For this review, take the finished solid that the model builds, in its own axes (mm). Give positions to 0.01 mm unless a question says otherwise; leave off trailing zeros. Write each loop counter-clockwise with the first axis right and the second up, starting at its lowest first coordinate (ties: lowest second). Pieces come first, ordered by that corner, then holes. Notation, with made-up numbers: M -22.75,-36 L 30.25,-36 A20 cw 30.25,-5 Z; hole C 44.5,84 d7. An arc over 180 degrees is marked long. One line per item, written item: value. Start each with the question number.
Item 1: To check wall thickness, follow probe 1 along X at (y, z) = (0.5, 0.25); probe 2 along X at (y, z) = (2.5, -1.25); probe 3 along Z at (x, y) = (46.99, 1.5). State the ranges of each line that lie inside material, in increasing order.
Item 2: Consider section A-A, the plane x = 46.99. Write out the cut boundary in (y, z).
Item 3: Mouldability with a two-part tool opening along Z and no side actions: class faces 1 (the face through (-1, 3, 6.35)), 2 (the face through (-50.775, 3.131, -1.192)), 3 (the face through (-1, 3, -6.35)) as released by +Z, released by -Z, zero draft, split by the parting line, or undercut.
Item 4: Consider section B-B, the plane z = 0. Write out the cut boundary in (x, y).
Item 5: Consider section C-C, the plane y = 1.5. Write out the cut boundary in (x, z), and give its area (3 significant figures).
```python
from build123d import *

# Parameters (mm, degrees)
SKETCH1_W                          = 114.3
SKETCH1_H                          = 12.7
BOSS_EXTRUDE1_DEPTH                = 6.35
F_5_16_0_3125_DIAMETER_HOLE1_D     = 7.9375
F_5_16_0_3125_DIAMETER_HOLE1_DEPTH = 14.986
F_5_16_0_3125_DIAMETER_HOLE1_TIP   = 2.384665582


with BuildPart() as part:
    # Sketch1 → Boss-Extrude1 (new body)
    with BuildSketch(Plane(origin=(0, 0, 0), x_dir=(1, 0, 0), z_dir=(0, 1, 0))):
        Rectangle(SKETCH1_W, SKETCH1_H)
    extrude(amount=BOSS_EXTRUDE1_DEPTH)

    # 5/16 (0.3125) Diameter Hole1
    with Locations(Plane(origin=(0, 6.35, 0), x_dir=(1, 0, 0), z_dir=(0, 1, 0))):
        with Locations((-46.99, 0), (46.99, 0)):
            Hole(F_5_16_0_3125_DIAMETER_HOLE1_D / 2, depth=F_5_16_0_3125_DIAMETER_HOLE1_DEPTH)
            with Locations((0, 0, -(F_5_16_0_3125_DIAMETER_HOLE1_DEPTH + F_5_16_0_3125_DIAMETER_HOLE1_TIP / 2))):  # 118° drill point
                Cone(0, F_5_16_0_3125_DIAMETER_HOLE1_D / 2, F_5_16_0_3125_DIAMETER_HOLE1_TIP, mode=Mode.SUBTRACT)


solid = part.part
```
Model answer:
1. probe 1: x = -57.15 to -50.95, -43.03 to 43.03, 50.95 to 57.15
1. probe 2: x = -57.15 to -50.76, -43.22 to 43.22, 50.76 to 57.15
1. probe 3: z = -6.35 to -3.97, 3.97 to 6.35
2. outline: M 0,-6.35 L 6.35,-6.35 L 6.35,-3.97 L 0,-3.97 Z; M 0,3.97 L 6.35,3.97 L 6.35,6.35 L 0,6.35 Z
3. face 1: released by +Z
3. face 2: undercut
3. face 3: released by -Z
4. outline: M -57.15,0 L -50.96,0 L -50.96,6.35 L -57.15,6.35 Z; M -43.02,0 L 43.02,0 L 43.02,6.35 L -43.02,6.35 Z; M 50.96,0 L 57.15,0 L 57.15,6.35 L 50.96,6.35 Z
5. outline: M -57.15,-6.35 L 57.15,-6.35 L 57.15,6.35 L -57.15,6.35 Z; hole C -46.99,0 d7.94; hole C 46.99,0 d7.94
5. area: 1,350 mm2
